Work out the finished part from the listing and answer in its coordinate system (mm). Face numbers are marked on the shaded views. A direction names the side the tool comes from. Round coordinates to 2 decimals unless told otherwise and drop trailing zeros. Order: outer loops, then holes, each group sorted by start corner. A loop starts at its lowest first (then second) coordinate and runs counter-clockwise, first axis right, second up. Notation, with made-up numbers: (-6.75, -24.75) -> (6.25, -24.75) arc R12 ccw to (6.25, -5.75) -> close; hole circle Ø7 at (26.25, -10). An arc over 180 degrees is marked (long way). Use a Markdown table: item, result. Add a question column.
Item 1: For a pull along X with two mould halves and no side action, classify the marked faces 4, 5 and 6 as +X half, -X half, draft (parallel to the pull), parting line (faces both ways), or undercut.
Item 2: Find the intervals of material crossed by L1, parallel to X at y = 2, z = -3 (3 decimals); L2, parallel to X at y = 19, z = 6 (3 decimals); L3, parallel to Z at x = 6, y = 14.5, in increasing order. Write a range as [from, to].
Item 3: A tool of negligible diameter and unlimited length cuts with its end or side. For the marked faces 1, 2 and 3, from which of +Z, -Z, +X, -X, +Y, -Y can it reach the whole face along a straight path? Write none if from no direction.
Item 4: A cutting plane is placed at A-A, the plane z = -6. Determine the outline of the cut face in (x, y) (3 decimals), plus the area to 3 significant figures.
Item 5: A cutting plane is placed at C-C, the plane y = 20. Determine the outline of the cut face in (x, z) (3 decimals).
Item 6: A cutting plane is placed at B-B, the plane z = 10. Determine the outline of the cut face in (x, y) (3 decimals), plus the area to 3 significant figures.
Item 7: A cutting plane is placed at D-D, the plane x = -2. Determine the outline of the cut face in (y, z), plus the area to 3 significant figures.
Item 8: A flat-ended cylindrical pin translates along its axis: P1, Ø4, axis at x = 19.66, z = -16.26, coming from the +Y side. Find the tip coordinate at first contact, or state that the pin passes through.
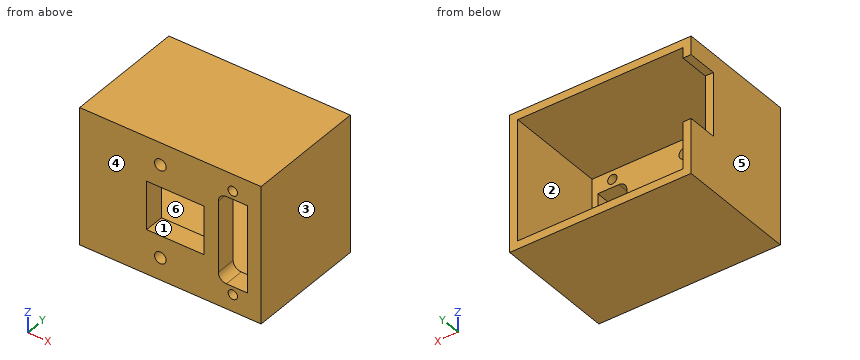
from build123d import *

# Parameters (mm, degrees)
SKETCH1_W             = 57.15
SKETCH1_H             = 43.18
BOSS_EXTRUDE1_DEPTH   = 38.1
SKETCH2_W             = 52.07
SKETCH2_H             = 38.1
CUT_EXTRUDE1_DEPTH    = 31.75
SKETCH3_W             = 18.034
SKETCH3_H             = 15.24
CUT_EXTRUDE2_DEPTH    = 53.290235465
CUT_EXTRUDE3_REACH    = 73.999
SKETCH4_W             = 20.066
SKETCH4_H             = 9.525
CUT_EXTRUDE4_REACH    = 54.29
F_4_CLEARANCE_HOLE1_D = 2.9464
F_6_CLEARANCE_HOLE1_D = 3.6576


with BuildPart() as part:
    # Sketch1 → Boss-Extrude1 (new body)
    with BuildSketch(Plane(origin=(0, 0, 0), x_dir=(1, 0, 0), z_dir=(0, 1, 0))):
        Rectangle(SKETCH1_W, SKETCH1_H)
    extrude(amount=BOSS_EXTRUDE1_DEPTH)

    # Sketch2 → Cut-Extrude1 (cut)
    with BuildSketch(Plane(origin=(0, 38.1, 0), x_dir=(1, 0, 0), z_dir=(0, 1, 0))):
        Rectangle(SKETCH2_W, SKETCH2_H)
    extrude(amount=-CUT_EXTRUDE1_DEPTH, mode=Mode.SUBTRACT)

    # Sketch3 → Cut-Extrude2 (cut, through all)
    with BuildSketch(Plane(origin=(0, 0, 0), x_dir=(-1, 0, 0), z_dir=(0, -1, 0))):
        with Locations((-1.524, 0)):
            Rectangle(SKETCH3_W, SKETCH3_H)
    extrude(amount=-CUT_EXTRUDE2_DEPTH, mode=Mode.SUBTRACT)

    # Sketch4 → Cut-Extrude3 (cut, up to next)
    with BuildSketch(Plane.ZY.offset(28.575), mode=Mode.PRIVATE) as cut_extrude3_sk1:
        with Locations((5.715, 33.3375)):
            Rectangle(SKETCH4_W, SKETCH4_H)
    cut_extrude3_tool1 = extrude(cut_extrude3_sk1.sketch, amount=-CUT_EXTRUDE3_REACH, mode=Mode.PRIVATE) & part.part
    add(cut_extrude3_tool1.solids().sort_by_distance((-28.575, 33.3375, 5.715))[0], mode=Mode.SUBTRACT)

    # Sketch5 → Cut-Extrude4 (cut, up to next)
    with BuildSketch(Plane.XZ, mode=Mode.PRIVATE) as cut_extrude4_sk1:
        with BuildLine():
            Line((17.624947543, -13.716), (24.228947543, -13.716))
            Line((24.228947543, -13.716), (24.228947543, 13.716))
            Line((24.228947543, 13.716), (17.624947543, 13.716))
            ThreePointArc((17.624947543, 13.716), (15.828896319, 12.972051224), (15.084947543, 11.176))
            Line((15.084947543, 11.176), (15.084947543, -11.176))
            ThreePointArc((15.084947543, -11.176), (15.828896319, -12.972051224), (17.624947543, -13.716))
        make_face()
    cut_extrude4_tool1 = extrude(cut_extrude4_sk1.sketch, amount=-CUT_EXTRUDE4_REACH, mode=Mode.PRIVATE) & part.part
    add(cut_extrude4_tool1.solids().sort_by_distance((19.701649, 0, 0))[0], mode=Mode.SUBTRACT)

    # #4 Clearance Hole1 (through all)
    with Locations(Plane(origin=(0, 0, 0), x_dir=(-1, 0, 0), z_dir=(0, -1, 0))):
        with Locations((-19.656947543, 16.256), (-19.656947543, -16.256)):
            Hole(F_4_CLEARANCE_HOLE1_D / 2)

    # #6 Clearance Hole1 (through all)
    with Locations(Plane(origin=(0, 0, 0), x_dir=(-1, 0, 0), z_dir=(0, -1, 0))):
        with Locations((3.175, 14.605), (3.175, -14.605)):
            Hole(F_6_CLEARANCE_HOLE1_D / 2)


solid = part.part
Reported:
| question | item | result |
|---|---|---|
| 1 | face 4 | draft |
| 1 | face 5 | -X half |
| 1 | face 6 | undercut |
| 2 | L1 | [-28.575, -7.493], [10.541, 15.085], [24.229, 28.575] |
| 2 | L2 | [-28.575, -26.035], [26.035, 28.575] |
| 2 | L3 | [-21.59, -19.05], [19.05, 21.59] |
| 3 | face 1 | +Y, -Y |
| 3 | face 2 | +Y |
| 3 | face 3 | +Z, -Z, +X, +Y, -Y |
| 4 | outline | (-28.575, 0) -> (-7.493, 0) -> (-7.493, 6.35) -> (-26.035, 6.35) -> (-26.035, 38.1) -> (-28.575, 38.1) -> close; (10.541, 0) -> (15.085, 0) -> (15.085, 6.35) -> (10.541, 6.35) -> close; (24.229, 0) -> (28.575, 0) -> (28.575, 38.1) -> (26.035, 38.1) -> (26.035, 6.35) -> (24.229, 6.35) -> close |
| 4 | area | 352 mm² |
| 5 | outline | (-28.575, -21.59) -> (28.575, -21.59) -> (28.575, 21.59) -> (-28.575, 21.59) -> close; hole (-26.035, -19.05) -> (26.035, -19.05) -> (26.035, 19.05) -> (-26.035, 19.05) -> close |
| 6 | outline | (-28.575, 0) -> (15.085, 0) -> (15.085, 6.35) -> (-26.035, 6.35) -> (-26.035, 28.575) -> (-28.575, 28.575) -> close; (24.229, 0) -> (28.575, 0) -> (28.575, 38.1) -> (26.035, 38.1) -> (26.035, 6.35) -> (24.229, 6.35) -> close |
| 6 | area | 442 mm² |
| 7 | outline | (0, -21.59) -> (38.1, -21.59) -> (38.1, -19.05) -> (6.35, -19.05) -> (6.35, -16.01) -> (0, -16.01) -> close; (0, -13.2) -> (6.35, -13.2) -> (6.35, -7.62) -> (0, -7.62) -> close; (0, 7.62) -> (6.35, 7.62) -> (6.35, 13.2) -> (0, 13.2) -> close; (0, 16.01) -> (6.35, 16.01) -> (6.35, 19.05) -> (38.1, 19.05) -> (38.1, 21.59) -> (0, 21.59) -> close |
| 7 | area | 303 mm² |
| 8 | P1 | y = 6.35 |
